Design review of the part built by this model. Coordinates are the model's own, in mm. Face numbers are marked on the shaded views. A direction names the side the tool comes from. Round coordinates to 2 decimals unless told otherwise and drop trailing zeros. Loops run counter-clockwise (first coordinate to the right, second up) from the corner with the lowest first, then second, coordinate; pieces in that order, holes last. Notation, with made-up numbers: M 33,-27.5 L 47,-27.5 A13 ccw 47,-16.5 Z; hole C 28,71.25 d3. An arc over 180 degrees is marked long. Answer as CSV lines item,"result". Start each with the question number.
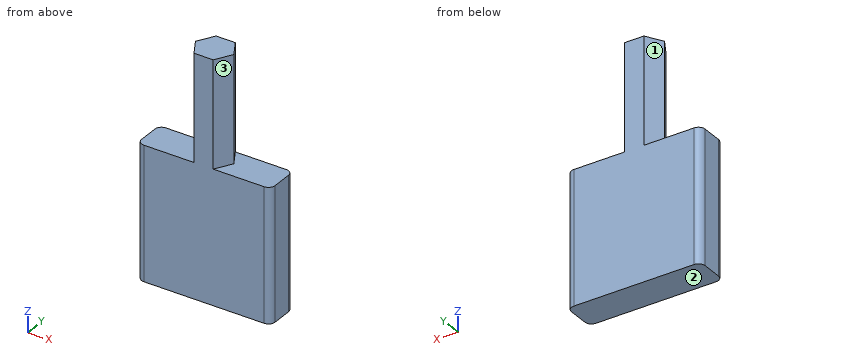
from build123d import *

# Parameters (mm, degrees)
F1_DEPTH      = 8
F2_W          = 10.055962
F2_H          = 10
F3_DEPTH      = 1.25
F3_DEPTH_BACK = 1.25
F4_R          = 0.5


with BuildPart() as f1:
    # F0 (on Top) → F1 (new body)
    with BuildSketch(Plane.XY):
        Polygon((0.721688, 1.25), (-0.721688, 1.25), (-1.443376, 0), (-0.721688, -1.25), (0.721688, -1.25), (1.443376, 0), align=None)
    extrude(amount=F1_DEPTH)

    # F2 (on Front) → F3 (join, two sides)
    with BuildSketch(Plane.XZ) as f3_sk:
        with Locations((0.027981, -5)):
            Rectangle(F2_W, F2_H)
    extrude(amount=F3_DEPTH)
    extrude(f3_sk.sketch, amount=-F3_DEPTH_BACK)

    # F4
    f4_edges = [f1.edges().sort_by_distance(p)[0] for p in [
        (5.055962, -1.25, -5),
        (5.055962, 1.25, -5),
        (-5, -1.25, -5),
        (-5, 1.25, -5),
    ]]
    fillet(f4_edges, radius=F4_R)


solid = f1.part
Item 1: Consider section B-B, the plane z = 6. Write out the cut boundary in (x, y), then the cut area to 3 significant figures.
Item 2: Consider section C-C, the plane x = 1.25. Write out the cut boundary in (y, z), then the cut area to 3 significant figures.
Item 3: Consider section D-D, the plane x = 3.75. Write out the cut boundary in (y, z), then the cut area to 3 significant figures.
Item 4: Tool access review of the marked faces 1, 2 and 3: name each direction out of +Z, -Z, +X, -X, +Y, -Y from which nothing blocks a thin tool from reaching the whole face with its end or side.
Item 5: To check wall thickness, follow line 1 (Z direction, x = 2, y = -0.1); line 2 (X direction, y = -0.4, z = 5.5); line 3 (X direction, y = 0.7, z = 1.75). State the ranges of each line that lie inside material, in increasing order.
Item 6: Consider section A-A, the plane x = -1. Write out the cut boundary in (y, z).
Found:
1,outline,"M -1.44,0 L -0.72,-1.25 L 0.72,-1.25 L 1.44,0 L 0.72,1.25 L -0.72,1.25 Z"
1,area,"5.41 mm^2"
2,outline,"M -1.25,-10 L 1.25,-10 L 1.25,0 L 0.33,0 L 0.33,8 L -0.33,8 L -0.33,0 L -1.25,0 Z"
2,area,"30.4 mm^2"
3,outline,"M -1.25,-10 L 1.25,-10 L 1.25,0 L -1.25,0 Z"
3,area,"25.0 mm^2"
4,face 1,"+Z, -X, +Y"
4,face 2,"-Z, +X, -X, +Y, -Y"
4,face 3,"+Z, +X, -Y"
5,line 1,"z = -10 to 0"
5,line 2,"x = -1.21 to 1.21"
5,line 3,"x = -1.04 to 1.04"
6,outline,"M -1.25,-10 L 1.25,-10 L 1.25,0 L 0.77,0 L 0.77,8 L -0.77,8 L -0.77,0 L -1.25,0 Z"
